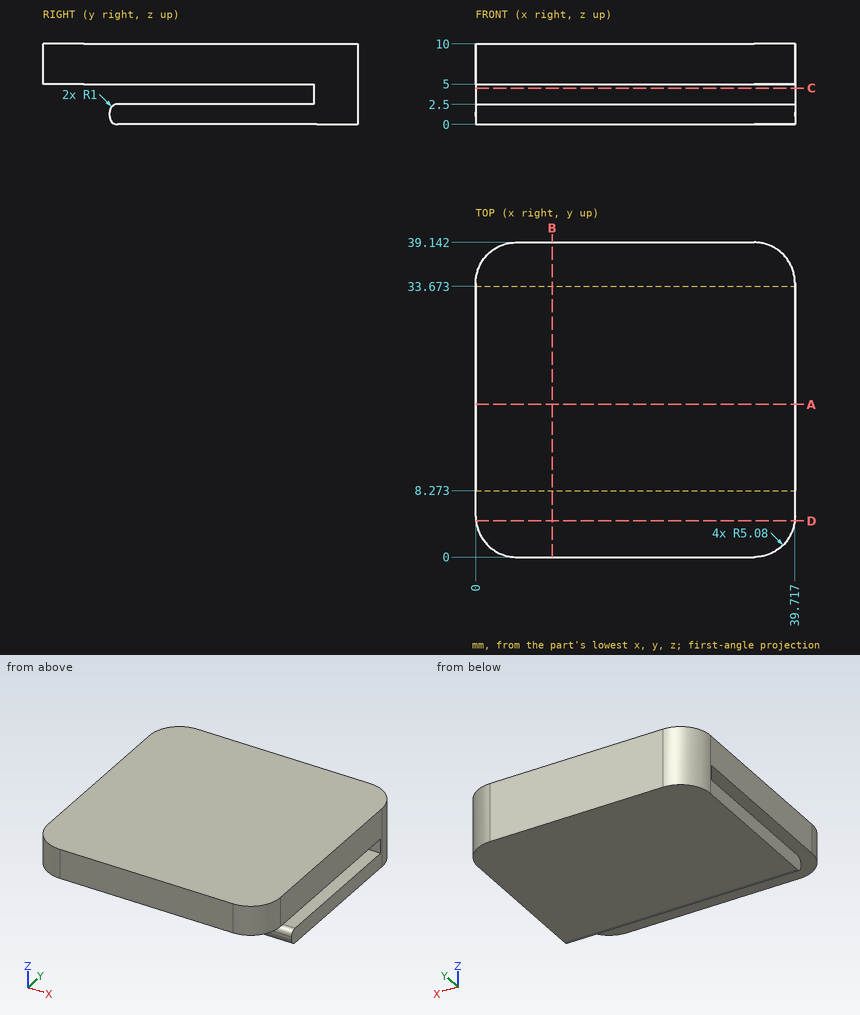
Study the drawing (mm; zero at the part's minimum x, y, z) and answer. Round coordinates to 2 decimals unless told otherwise and drop trailing zeros. Write each loop counter-clockwise with the first axis right and the second up, starting at its lowest first coordinate (ties: lowest second). Pieces come first, ordered by that corner, then holes.
1) A cutting plane is placed at C-C on z = 4.5. Determine the outline of the cut face in (x, y), and give its area (3 significant figures).
2) A cutting plane is placed at A-A on y = 19. Determine the outline of the cut face in (x, z), and give its area (3 significant figures).
3) A cutting plane is placed at B-B on x = 9.5. Determine the outline of the cut face in (y, z).
4) Consider probe 1 along Z at (x, y) = (27, 17); probe 2 along Y at (x, z) = (25, 4); probe 3 along Y at (x, z) = (28.5, 1.5). Determine where each line is inside the solid, lowest interval first.
5) A cutting plane is placed at D-D on y = 4.5. Determine the outline of the cut face in (x, z), and give its area (3 significant figures).
Entries:
1. outline: (0, 33.67) - (39.72, 33.67) - (39.72, 34.06) arc R5.08 ccw to (34.64, 39.14) - (5.08, 39.14) arc R5.08 ccw to (0, 34.06) - close
1. area: 206 mm2
2. outline: (0, 0) - (39.72, 0) - (39.72, 2.5) - (0, 2.5) - close; (0, 5) - (39.72, 5) - (39.72, 10) - (0, 10) - close
2. area: 298 mm2
3. outline: (0, 5) - (33.67, 5) - (33.67, 2.5) - (9.27, 2.5) arc R1 ccw to (8.27, 1.5) - (8.27, 1) arc R1 ccw to (9.27, 0) - (39.14, 0) - (39.14, 10) - (0, 10) - close
4. probe 1: z = 0 to 2.5, 5 to 10
4. probe 2: y = 33.67 to 39.14
4. probe 3: y = 8.27 to 39.14
5. outline: (0.03, 5) - (39.68, 5) - (39.68, 10) - (0.03, 10) - close
5. area: 198 mm2
